Could you check a few things on this drawing? It's one solid part, dimensions in mm from its lowest x, y, z. A direction names the side the tool comes from. Give positions to 0.01 mm unless a question says otherwise; leave off trailing zeros. Loops run counter-clockwise (first coordinate to the right, second up) from the corner with the lowest first, then second, coordinate; pieces in that order, holes last. Notation, with made-up numbers: (18.25, -4) - (63.25, -4) arc R6 cw to (63.25, 2) - close; hole circle Ø10 at (63.5, 62.25). An arc over 180 degrees is marked (long way). Answer as a JSON object with one key per item and string values.
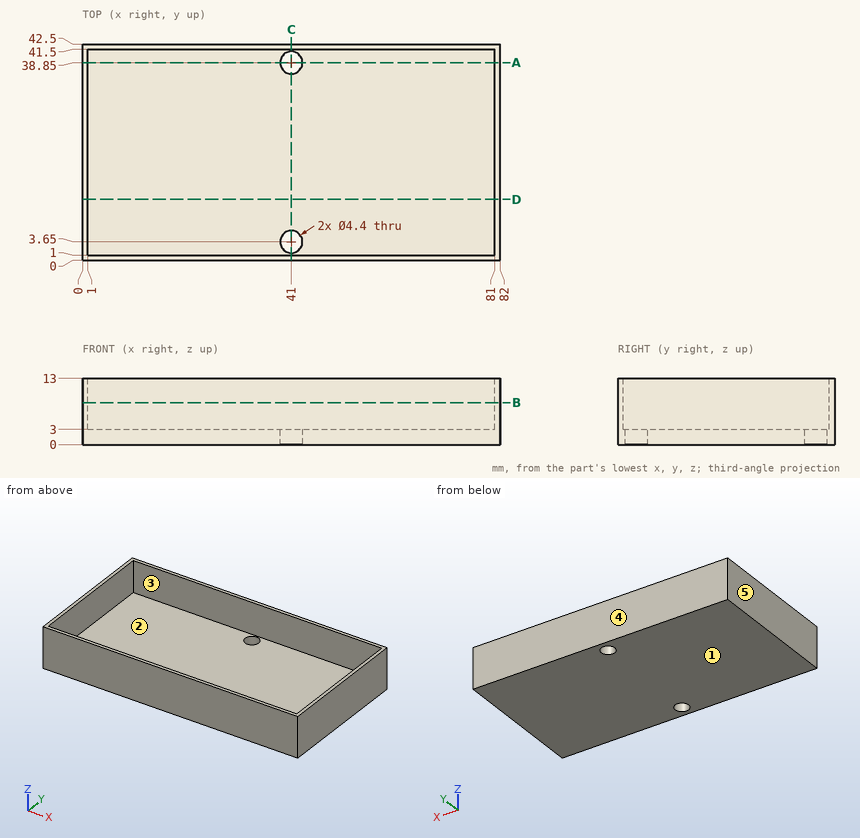
1) Imagine slicing it at D-D on y = 12. Write out the boundary of the cut face in (x, z), and give its area (3 significant figures).
Check sheet entries:
{"outline": "(0, 0) - (82, 0) - (82, 13) - (81, 13) - (81, 3) - (1, 3) - (1, 13) - (0, 13) - close", "area": "266 mm2"}
2) I'm going to push flat-ended pins straight in: P1, Ø5, axis at y = 26.5, z = 9, coming from the -X side; P2, Ø6, axis at x = 65.5, y = 13, coming from the +Z side. Where does each tip first touch, or does it pass through?
Check sheet entries:
{"P1": "x = 0", "P2": "z = 3"}
3) Which directions (+Z, -Z, +X, -X, +Y, -Y) give clear straight access to the entire face, cutting with the end or side of a thin tool? Please do the marked faces 1 and 2.
Check sheet entries:
{"face 1": "-Z, +X, -X, +Y, -Y", "face 2": "+Z"}
4) If we mould it in two halves opening along Y, with no side actions, what happens to the marked faces 3, 4 and 5? For each: released by +Y, released by -Y, zero draft, split by the parting line, or undercut.
Check sheet entries:
{"face 3": "undercut", "face 4": "released by +Y", "face 5": "zero draft"}
5) Imagine slicing it at C-C on x = 41. Write out the boundary of the cut face in (y, z).
Check sheet entries:
{"outline": "(0, 0) - (1.45, 0) - (1.45, 3) - (1, 3) - (1, 13) - (0, 13) - close; (5.85, 0) - (36.65, 0) - (36.65, 3) - (5.85, 3) - close; (41.05, 0) - (42.5, 0) - (42.5, 13) - (41.5, 13) - (41.5, 3) - (41.05, 3) - close"}
6) Imagine slicing it at A-A on y = 38.85. Write out the boundary of the cut face in (x, z).
Check sheet entries:
{"outline": "(0, 0) - (38.8, 0) - (38.8, 3) - (1, 3) - (1, 13) - (0, 13) - close; (43.2, 0) - (82, 0) - (82, 13) - (81, 13) - (81, 3) - (43.2, 3) - close"}
7) Imagine slicing it at B-B on z = 8.25. Write out the boundary of the cut face in (x, y).
Check sheet entries:
{"outline": "(0, 0) - (82, 0) - (82, 42.5) - (0, 42.5) - close; hole (1, 1) - (81, 1) - (81, 41.5) - (1, 41.5) - close"}
8) I need wall thicknesses on L1, parallel to Y at x = 41, z = 2.1; L2, parallel to Y at x = 40, z = 8.75; L3, parallel to X at y = 18, z = 12. Which ranges of each line are inside material? Lowest first, please.
Check sheet entries:
{"L1": "0 to 1.45, 5.85 to 36.65, 41.05 to 42.5", "L2": "0 to 1, 41.5 to 42.5", "L3": "0 to 1, 81 to 82"}
